from build123d import *

# Parameters (mm, degrees)
SKETCH1_R           = 2.025
SKETCH1_R_2         = 2
BOSS_EXTRUDE1_DEPTH = 3
BOSS_EXTRUDE2_DEPTH = 3
SKETCH3_R           = 1.5
CUT_EXTRUDE1_DEPTH  = 323.081088677


with BuildPart() as part:
    # Sketch1 → Boss-Extrude1 (new body)
    with BuildSketch(Plane.XY):
        Polygon((-22.319441397, -137.107072194), (-30.931230202, -145.718860999), (-30.931230202, -211.799971874), (-15.316322, -227.735842242), (14.74833584, -227.638274393), (227.638274393, -14.74833584), (227.735842242, 15.316322), (211.799971874, 30.931230202), (145.718860999, 30.931230202), (137.107072194, 22.319441397), (137.107072194, -34.003174495), (34.003174495, -137.107072194), align=None)
        with Locations((-22.931230202, -167.944306144)):
            Circle(SKETCH1_R, mode=Mode.SUBTRACT)
        with Locations((7.068769798, -167.944306144)):
            Circle(SKETCH1_R, mode=Mode.SUBTRACT)
        with Locations((-22.931230202, -145.107072194)):
            Circle(SKETCH1_R, mode=Mode.SUBTRACT)
        with Locations((7.068769798, -145.107072194)):
            Circle(SKETCH1_R, mode=Mode.SUBTRACT)
        with Locations((71.929470696, -139.81172169)):
            Circle(SKETCH1_R, mode=Mode.SUBTRACT)
        with Locations((55.781107706, -123.6633587)):
            Circle(SKETCH1_R, mode=Mode.SUBTRACT)
        with Locations((167.944306144, 22.931230202)):
            Circle(SKETCH1_R, mode=Mode.SUBTRACT)
        with Locations((139.81172169, -71.929470696)):
            Circle(SKETCH1_R, mode=Mode.SUBTRACT)
        with Locations((145.107072194, -7.068769798)):
            Circle(SKETCH1_R, mode=Mode.SUBTRACT)
        with Locations((145.107072194, 22.931230202)):
            Circle(SKETCH1_R, mode=Mode.SUBTRACT)
        with Locations((167.944306144, -7.068769798)):
            Circle(SKETCH1_R, mode=Mode.SUBTRACT)
        with Locations((123.6633587, -55.781107706)):
            Circle(SKETCH1_R_2, mode=Mode.SUBTRACT)
    extrude(amount=BOSS_EXTRUDE1_DEPTH)

    # Sketch2 → Boss-Extrude2 (add)
    with BuildSketch(Plane.XY.offset(3)):
        with BuildLine():
            Line((66.463240253, -48.078463942), (48.078463942, -66.463240253))
            ThreePointArc((48.078463942, -66.463240253), (46.613997848, -69.998774159), (48.078463942, -73.534308065))
            Line((48.078463942, -73.534308065), (69.291667378, -94.7475115))
            ThreePointArc((69.291667378, -94.7475115), (70.756133472, -98.283045406), (69.291667378, -101.818579312))
            Line((69.291667378, -101.818579312), (72.827201283, -98.283045406))
            Line((72.827201283, -98.283045406), (85.555123345, -85.555123345))
            Line((85.555123345, -85.555123345), (98.283045406, -72.827201283))
            Line((98.283045406, -72.827201283), (101.818579312, -69.291667378))
            ThreePointArc((101.818579312, -69.291667378), (98.283045406, -70.756133472), (94.7475115, -69.291667378))
            Line((94.7475115, -69.291667378), (73.534308065, -48.078463942))
            ThreePointArc((73.534308065, -48.078463942), (69.998774159, -46.613997848), (66.463240253, -48.078463942))
        make_face()
    extrude(amount=-BOSS_EXTRUDE2_DEPTH)

    # Sketch3 → Cut-Extrude1 (cut, through all)
    with BuildSketch(Plane.XY.offset(3)):
        with Locations((49.744824715, -70.173841205)):
            Circle(SKETCH3_R)
        with Locations((89.342804461, -70.173841205)):
            Circle(SKETCH3_R)
        with BuildLine():
            Line((66.95938056, -87.220709483), (71.202021247, -91.46335017))
            ThreePointArc((71.202021247, -91.46335017), (72.61623481, -92.049136607), (74.030448372, -91.46335017))
            Line((74.030448372, -91.46335017), (81.808622965, -83.685175577))
            ThreePointArc((81.808622965, -83.685175577), (82.394409403, -82.270962014), (81.808622965, -80.856748452))
            Line((81.808622965, -80.856748452), (77.565982278, -76.614107765))
            ThreePointArc((77.565982278, -76.614107765), (76.151768716, -76.028321327), (74.737555153, -76.614107765))
            Line((74.737555153, -76.614107765), (66.95938056, -84.392282358))
            ThreePointArc((66.95938056, -84.392282358), (66.373594123, -85.80649592), (66.95938056, -87.220709483))
        make_face()
    extrude(amount=-CUT_EXTRUDE1_DEPTH, mode=Mode.SUBTRACT)


solid = part.part
Here's how the part is built. I have some questions about the finished solid (model axes, mm). A direction names the side the tool comes from. Round coordinates to 2 decimals unless told otherwise and drop trailing zeros. Order: outer loops, then holes, each group sorted by start corner. A loop starts at its lowest first (then second) coordinate and runs counter-clockwise, first axis right, second up. Notation, with made-up numbers: M 25,-12.75 L 74,-12.75 A15 cw 74,13.25 Z; hole C 49.5,32 d5. An arc over 180 degrees is marked long. Return JSON: item names as keys, results as strings. Group by question number.
1. Please list where these lines run through material, in increasing order: probe 1 along X at (y, z) = (-146, 1.55); probe 2 along X at (y, z) = (-143.5, 2); probe 3 along X at (y, z) = (-69, 1.8).
2. If we mould it in two halves opening along X, with no side actions, what happens to faces 1 (the face through (98, -98, 3)), 2 (the face through (219.879, 23.014, 1.479)), 3 (the face through (70.9, -80.45, 1.52)), 4 (the face through (58.537, -83.992, 1.521))? For each: pulls with the +X half, pulls with the -X half, needs draft (parallel to the pull), parting line crosses it, or undercut.
3. I'm going to push flat-ended pins straight in: pin 1 Ø6.5 at (x, y) = (55.78, -123.66) entering from +Z; pin 2 Ø1.5 at (y, z) = (-181, 0.5) entering from +X; pin 3 Ø1.5 at (y, z) = (-7.5, 1) entering from -X; pin 4 Ø0.9 at (x, z) = (-3, 1.5) entering from +Y. Where does each tip first touch, or does it pass through?
4. If we section it at B-B on y = -39: List the corners of the cut face in (x, z) for me.
5. If we section it at A-A on x = 183: List the corners of the cut face in (y, z) for me, then the cut area to 3 significant figures.
6. If we section it at C-C on z = 1.1: State how many separate pieces and enclosed holes the cut face has, then the cut area to 3 significant figures.
7. On a 3-axis mill with a long thin cutter (end or side, diameter ignored), from which of +Z, -Z, +X, -X, +Y, -Y can I reach the whole of each face in a straight line? I mean faces 5 (the face through (84.289, -58.834, 1.521)), 6 (the face through (51.89, -119.22, 1.48)), 7 (the face through (77.865, -87.629, 1.521)). Say none if no direction works.
Reply:
{
 "1": {"probe 1": "-30.93 to -24.75, -21.11 to 5.25, 8.89 to 96.39", "probe 2": "-28.71 to -24.16, -21.7 to 5.84, 8.3 to 98.89", "probe 3": "46.71 to 48.81, 50.68 to 88.41, 90.28 to 94.46, 102.11 to 173.39"},
 "2": {"face 1": "needs draft", "face 2": "pulls with the +X half", "face 3": "undercut", "face 4": "pulls with the -X half"},
 "3": {"pin 1": "z = 3", "pin 2": "x = 62.14", "pin 3": "x = 137.11", "pin 4": "y = -137.11"},
 "4": {"outline": "M 132.11,0 L 203.39,0 L 203.39,3 L 132.11,3 Z"},
 "5": {"outline": "M -59.39,0 L 30.93,0 L 30.93,3 L -59.39,3 Z", "area": "271 mm^2"},
 "6": {"separate pieces": "1", "enclosed holes": "15", "area": "22,100 mm^2"},
 "7": {"face 5": "+Z, -Z, +Y", "face 6": "+Z, -Z, -X", "face 7": "+Z, -Z"}
}
